Can you work these out from the drawing? Everything is in mm from the part's minimum corner. A direction names the side the tool comes from. Round coordinates to 2 decimals unless told otherwise and drop trailing zeros. Order: outer loops, then holes, each group sorted by start corner. A loop starts at its lowest first (then second) coordinate and runs counter-clockwise, first axis right, second up. Notation, with made-up numbers: (-5.5, 38.25) -> (24.5, 38.25) arc R28 ccw to (24.5, 56.25) -> close; hole circle Ø10 at (32.25, -2.75). An arc over 180 degrees is marked (long way). Use a Markdown table: item, result. Add a question column.
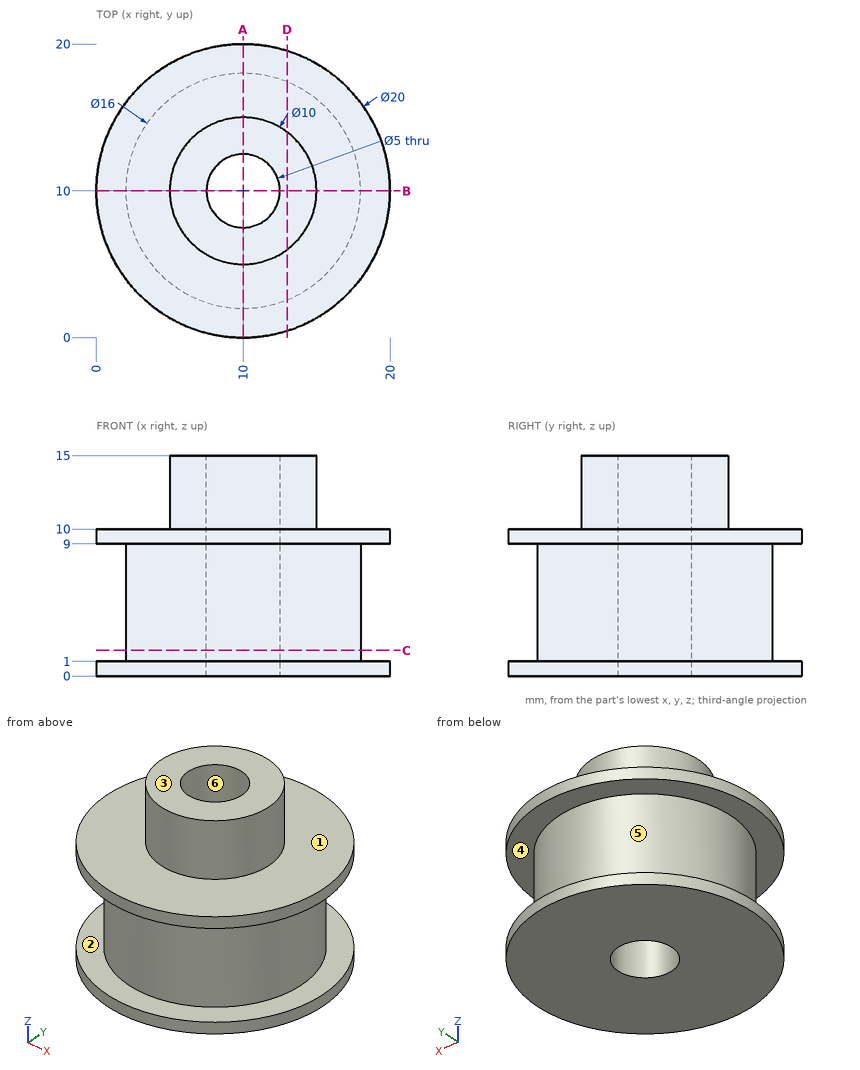
(1) I want a section at D-D on x = 13. List the corners of the cut face in (y, z) for me, and give its area (3 significant figures).
(2) I'm going to push flat-ended pins straight in: P1, Ø1, axis at x = 11.5, z = 3, coming from the +Y side; P2, Ø8, axis at y = 18, z = 9.5, coming from the -X side; P3, Ø4.5, axis at x = 10, y = 10, coming from the -Z side; P4, Ø4, axis at x = 14.5, y = 17, coming from the +Z side. Where does each tip first touch, or does it pass through?
(3) Please list where these lines run through material, in increasing order: probe 1 along Z at (x, y) = (6.5, 1); probe 2 along Y at (x, z) = (10, 6.5); probe 3 along Y at (x, z) = (10, 11). Write a range as from..to.
(4) I want a section at A-A on x = 10. List the corners of the cut face in (y, z) for me.
(5) If we mould it in two halves opening along X, with no side actions, what happens to the marked faces 4, 5 and 6? For each: pulls with the +X half, pulls with the -X half, needs draft (parallel to the pull), parting line crosses it, or undercut.
(6) I want a section at C-C on z = 1.75. List the corners of the cut face in (x, y) for me, and give its area (3 significant figures).
(7) On a 3-axis mill with a long thin cutter (end or side, diameter ignored), from which of +Z, -Z, +X, -X, +Y, -Y can I reach the whole of each face in a straight line? I mean the marked faces 1, 2 and 3. Say none if no direction works.
Output:
| question | item | result |
|---|---|---|
| 1 | outline | (0.46, 0) -> (19.54, 0) -> (19.54, 1) -> (17.42, 1) -> (17.42, 9) -> (19.54, 9) -> (19.54, 10) -> (14, 10) -> (14, 15) -> (6, 15) -> (6, 10) -> (0.46, 10) -> (0.46, 9) -> (2.58, 9) -> (2.58, 1) -> (0.46, 1) -> close |
| 1 | area | 197 mm² |
| 2 | P1 | y = 17.94 |
| 2 | P2 | x = 0.83 |
| 2 | P3 | through |
| 2 | P4 | z = 10 |
| 3 | probe 1 | 0..1, 9..10 |
| 3 | probe 2 | 2..7.5, 12.5..18 |
| 3 | probe 3 | 5..7.5, 12.5..15 |
| 4 | outline | (0, 0) -> (7.5, 0) -> (7.5, 15) -> (5, 15) -> (5, 10) -> (0, 10) -> (0, 9) -> (2, 9) -> (2, 1) -> (0, 1) -> close; (12.5, 0) -> (20, 0) -> (20, 1) -> (18, 1) -> (18, 9) -> (20, 9) -> (20, 10) -> (15, 10) -> (15, 15) -> (12.5, 15) -> close |
| 5 | face 4 | needs draft |
| 5 | face 5 | parting line crosses it |
| 5 | face 6 | undercut |
| 6 | outline | circle Ø16 at (10, 10); hole circle Ø5 at (10, 10) |
| 6 | area | 181 mm² |
| 7 | face 1 | +Z |
| 7 | face 2 | none |
| 7 | face 3 | +Z, +X, -X, +Y, -Y |
